Could you check a few things on this drawing? It's one solid part, dimensions in mm from its lowest x, y, z. A direction names the side the tool comes from. Give positions to 0.01 mm unless a question says otherwise; leave off trailing zeros. Order: outer loops, then holes, each group sorted by start corner. A loop starts at its lowest first (then second) coordinate and runs counter-clockwise, first axis right, second up.
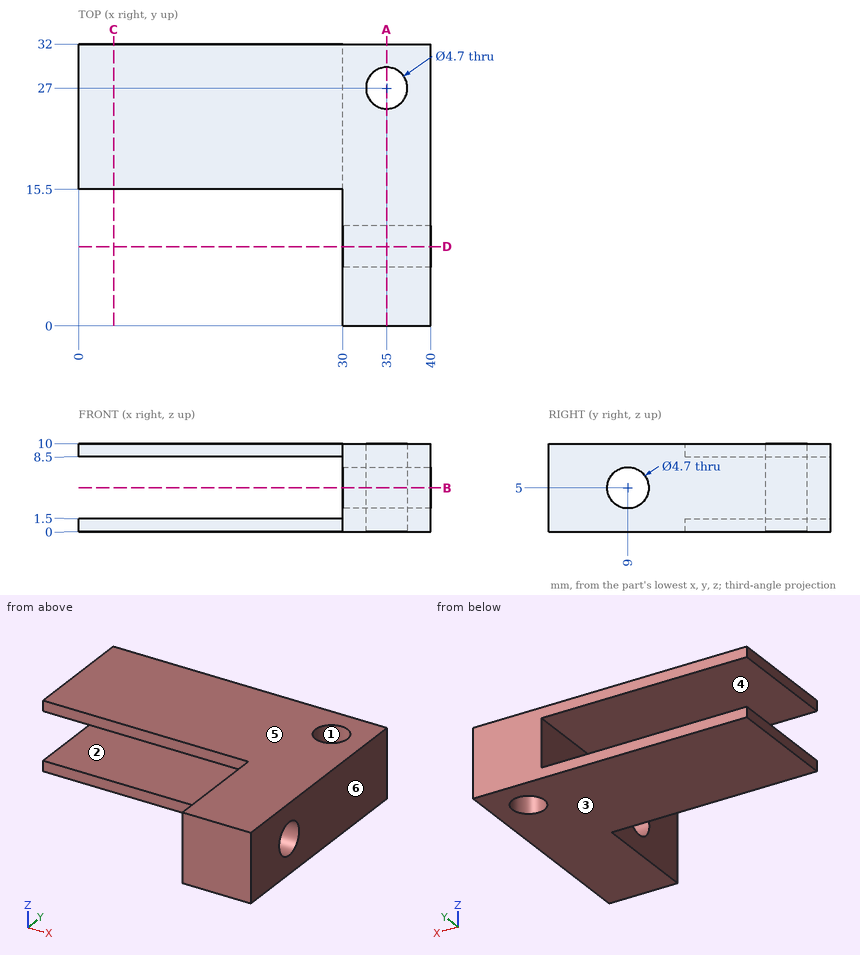
Item 1: Imagine slicing it at D-D on y = 9. List the corners of the cut face in (x, z) for me.
Findings:
outline: (30, 0) - (40, 0) - (40, 2.65) - (30, 2.65) - close; (30, 7.35) - (40, 7.35) - (40, 10) - (30, 10) - close
Item 2: Please list where these lines run through material, in increasing order: line 1 along Y through (x, z) = (35, 5); line 2 along Y through (x, z) = (36.5, 5); line 3 along Z through (x, y) = (9.5, 25.5).
Findings:
line 1: y = 0 to 6.65, 11.35 to 24.65, 29.35 to 32
line 2: y = 0 to 6.65, 11.35 to 25.19, 28.81 to 32
line 3: z = 0 to 1.5, 8.5 to 10
Item 3: Imagine slicing it at C-C on x = 4. List the corners of the cut face in (y, z) for me, then the cut area to 3 significant figures.
Findings:
outline: (15.5, 0) - (32, 0) - (32, 1.5) - (15.5, 1.5) - close; (15.5, 8.5) - (32, 8.5) - (32, 10) - (15.5, 10) - close
area: 49.5 mm2
Item 4: For pin 1 (1.2 mm diameter, centred on x = 11, z = 9, fed in from -Y), with a flat end and sliding along its axis, tell me the tip position at first contact or that it passes through.
Findings:
pin 1: stops at y = 15.5
Item 5: Imagine slicing it at B-B on z = 5. List the corners of the cut face in (x, y) for me, then the cut area to 3 significant figures.
Findings:
outline: (30, 0) - (40, 0) - (40, 6.65) - (30, 6.65) - close; (30, 11.35) - (40, 11.35) - (40, 32) - (30, 32) - close; hole circle Ø4.7 at (35, 27)
area: 256 mm2
Item 6: Imagine slicing it at A-A on x = 35. List the corners of the cut face in (y, z) for me, then the cut area to 3 significant figures.
Findings:
outline: (0, 0) - (24.65, 0) - (24.65, 10) - (0, 10) - close; (29.35, 0) - (32, 0) - (32, 10) - (29.35, 10) - close; hole circle Ø4.7 at (9, 5)
area: 256 mm2
Item 7: For the marked faces 1 and 2, which set-ups out of +Z, -Z, +X, -X, +Y, -Y let a thin tool reach every point of the face, with its end or its side?
Findings:
face 1: +Z, -Z
face 2: -X, +Y, -Y
Item 8: We'd pull the mould along Z, two halves only. Please class the marked faces 3, 4, 5 and 6: +Z half, -Z half, draft (parallel to the pull), parting line (faces both ways), or undercut.
Findings:
face 3: -Z half
face 4: undercut
face 5: +Z half
face 6: draft
